Here's the drawing with two shaded views (mm, measured from the low corner). I have some questions. Round coordinates to 2 decimals unless told otherwise and drop trailing zeros. Write each loop counter-clockwise with the first axis right and the second up, starting at its lowest first coordinate (ties: lowest second). Pieces come first, ordered by that corner, then holes. Notation, with made-up numbers: M 19.25,75 L 77.25,75 A26 ccw 77.25,91 Z; hole C 46.5,23.5 d3. An arc over 180 degrees is marked long. Answer as a JSON object with one key per item and string values. Group by question number.
1) If we mould it in two halves opening along X, with no side actions, what happens to the marked faces 1, 2, 3 and 4? For each: +X half, -X half, draft (parallel to the pull), parting line (faces both ways), or undercut.
2) Suppose I cut it at D-D, the plane z = 33.5. Write out the boundary of the cut face in (x, y).
3) Suppose I cut it at C-C, the plane x = 6. Write out the boundary of the cut face in (y, z) (1 decimal).
4) Suppose I cut it at B-B, the plane y = 3.1. Write out the boundary of the cut face in (x, z) (1 decimal).
5) I'm going to push flat-ended pins straight in: pin 1 Ø1.5 at (y, z) = (2, 13) entering from -X; pin 2 Ø1.5 at (y, z) = (3, 30) entering from -X; pin 3 Ø4 at (x, z) = (6, 14.36) entering from -Y; pin 4 Ø10 at (x, z) = (49, 10) entering from -Y. Where does each tip first touch, or does it pass through?
6) Suppose I cut it at A-A, the plane x = 41. Write out the boundary of the cut face in (y, z) (1 decimal).
7) Please list where these lines run through material, in increasing order: L1, parallel to X at y = 1.8, z = 14.5 (1 decimal); L2, parallel to Z at x = 57.5, y = 2.1 (1 decimal); L3, parallel to Z at x = 36.5, y = 1.6 (1 decimal). Write a range as [from, to].
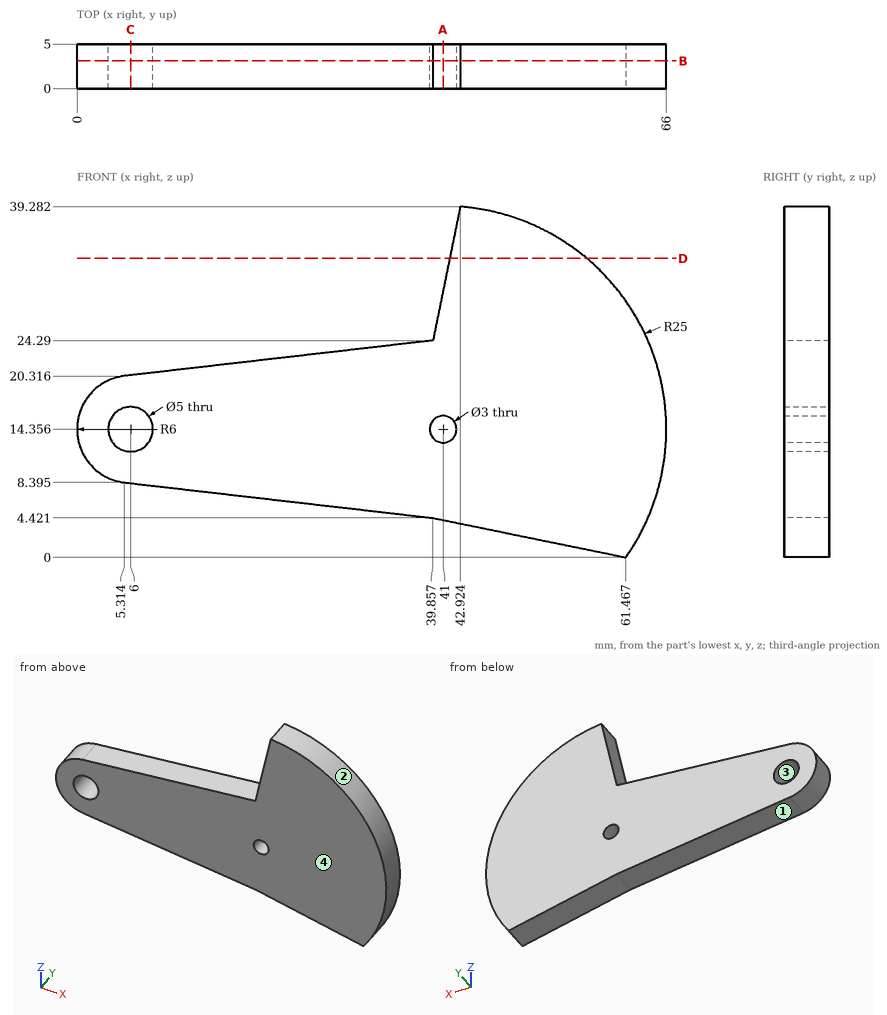
Results:
{
 "1": {"face 1": "-X half", "face 2": "+X half", "face 3": "undercut", "face 4": "draft"},
 "2": {"outline": "M 41.74,0 L 57.08,0 L 57.08,5 L 41.74,5 Z"},
 "3": {"outline": "M 0,8.3 L 5,8.3 L 5,11.9 L 0,11.9 Z; M 0,16.9 L 5,16.9 L 5,20.4 L 0,20.4 Z"},
 "4": {"outline": "M 5.3,8.4 L 39.9,4.4 L 61.5,0 A25 ccw 42.9,39.3 L 39.9,24.3 L 5.3,20.3 A6 ccw Z; hole C 6,14.4 d5; hole C 41,14.4 d3"},
 "5": {"pin 1": "x = 0.03", "pin 2": "x = 40.87", "pin 3": "through", "pin 4": "y = 0"},
 "6": {"outline": "M 0,4.2 L 5,4.2 L 5,12.9 L 0,12.9 Z; M 0,15.9 L 5,15.9 L 5,29.9 L 0,29.9 Z"},
 "7": {"L1": "[0, 3.5], [8.5, 39.5], [42.5, 66]", "L2": "[0.8, 33.1]", "L3": "[4.8, 23.9]"}
}
